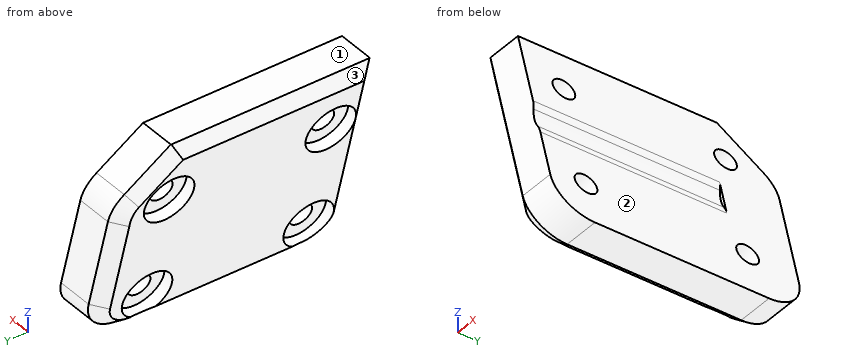
from build123d import *

# Parameters (mm, degrees)
CYLINDER119_R               = 2
CYLINDER119_DEPTH           = 1
CYLINDER119_PLACEMENT_ANGLE = 75
CYLINDER121_R               = 2
CYLINDER121_DEPTH           = 1
CYLINDER121_PLACEMENT_ANGLE = 75
CYLINDER122_R               = 2
CYLINDER122_DEPTH           = 1.4
CYLINDER122_PLACEMENT_ANGLE = 75
CYLINDER120_R               = 2
CYLINDER120_DEPTH           = 1.4
CYLINDER120_PLACEMENT_ANGLE = 75
CYLINDER118_R               = 2.4
CYLINDER118_DEPTH           = 15
CYLINDER118_ROLL_ANGLE      = 90
CYLINDER116_R               = 0.9
CYLINDER116_DEPTH           = 9
CYLINDER116_PLACEMENT_ANGLE = 75
CYLINDER117_R               = 0.9
CYLINDER117_DEPTH           = 9
CYLINDER117_PLACEMENT_ANGLE = 75
CYLINDER115_R               = 0.9
CYLINDER115_DEPTH           = 9
CYLINDER115_PLACEMENT_ANGLE = 75
CYLINDER114_R               = 0.9
CYLINDER114_DEPTH           = 9
CYLINDER114_PLACEMENT_ANGLE = 75
BOX098_W                    = 40
BOX098_H                    = 156
BOX098_DEPTH                = 130
BOX098_PITCH_ANGLE          = -15
BOX099_W                    = 30
BOX099_H                    = 156
BOX099_DEPTH                = 130
BOX099_PITCH_ANGLE          = -15
BOX100_W                    = 10
BOX100_H                    = 20
BOX100_DEPTH                = 16
CHAMFER010_SIZE             = 4
FILLET024_R                 = 3
CHAMFER011_SIZE             = 1
FILLET025_R                 = 2


with BuildPart() as cylinder119:
    # Cylinder119 → Cylinder119 (new body)
    with BuildSketch(Plane.XY):
        Circle(CYLINDER119_R)
    extrude(amount=CYLINDER119_DEPTH)


with BuildPart() as cylinder119_1:
    # Cylinder119 placement: moved
    add(cylinder119.part.moved(Location((509, -34, 102.5))).rotate(Axis((509, -34, 102.5), (0, 1, 0)), CYLINDER119_PLACEMENT_ANGLE))


with BuildPart() as fusion122:
    # Cylinder121 → Cylinder121 (new body)
    with BuildSketch(Plane.XY):
        Circle(CYLINDER121_R)
    extrude(amount=CYLINDER121_DEPTH)


with BuildPart() as fusion122_1:
    # Cylinder121 placement: moved
    add(fusion122.part.moved(Location((509, -21, 102.5))).rotate(Axis((509, -21, 102.5), (0, 1, 0)), CYLINDER121_PLACEMENT_ANGLE))

    # Fusion122: union Cylinder119
    add(cylinder119_1.part)


with BuildPart() as cylinder122:
    # Cylinder122 → Cylinder122 (new body)
    with BuildSketch(Plane.XY):
        Circle(CYLINDER122_R)
    extrude(amount=CYLINDER122_DEPTH)


with BuildPart() as cylinder122_1:
    # Cylinder122 placement: moved
    add(cylinder122.part.moved(Location((509, -34, 102.5))).rotate(Axis((509, -34, 102.5), (0, 1, 0)), CYLINDER122_PLACEMENT_ANGLE))


with BuildPart() as fusion123:
    # Cylinder120 → Cylinder120 (new body)
    with BuildSketch(Plane.XY):
        Circle(CYLINDER120_R)
    extrude(amount=CYLINDER120_DEPTH)


with BuildPart() as fusion123_1:
    # Cylinder120 placement: moved
    add(fusion123.part.moved(Location((509, -21, 102.5))).rotate(Axis((509, -21, 102.5), (0, 1, 0)), CYLINDER120_PLACEMENT_ANGLE))

    # Fusion124: union Cylinder122
    add(cylinder122_1.part)


with BuildPart() as fusion123_2:
    # Fusion124 placement: moved
    add(fusion123_1.part.moved(Location((2, 0, -9))))

    # Fusion123: union Fusion122
    add(fusion122_1.part)


with BuildPart() as cylinder118:
    # Cylinder118 → Cylinder118 (new body)
    with BuildSketch(Plane.XY):
        Circle(CYLINDER118_R)
    extrude(amount=CYLINDER118_DEPTH)


with BuildPart() as cylinder118_1:
    # Cylinder118 roll: moved
    add(cylinder118.part.rotate(Axis((0, 0, 0), (1, 0, 0)), CYLINDER118_ROLL_ANGLE))


with BuildPart() as cylinder118_2:
    # Cylinder118 placement: moved
    add(cylinder118_1.part.moved(Location((516, -22, 100))))


with BuildPart() as cylinder116:
    # Cylinder116 → Cylinder116 (new body)
    with BuildSketch(Plane.XY):
        Circle(CYLINDER116_R)
    extrude(amount=CYLINDER116_DEPTH)


with BuildPart() as cylinder116_1:
    # Cylinder116 placement: moved
    add(cylinder116.part.moved(Location((509, -34, 102.5))).rotate(Axis((509, -34, 102.5), (0, 1, 0)), CYLINDER116_PLACEMENT_ANGLE))


with BuildPart() as fusion120:
    # Cylinder117 → Cylinder117 (new body)
    with BuildSketch(Plane.XY):
        Circle(CYLINDER117_R)
    extrude(amount=CYLINDER117_DEPTH)


with BuildPart() as fusion120_1:
    # Cylinder117 placement: moved
    add(fusion120.part.moved(Location((509, -21, 102.5))).rotate(Axis((509, -21, 102.5), (0, 1, 0)), CYLINDER117_PLACEMENT_ANGLE))

    # Fusion120: union Cylinder116
    add(cylinder116_1.part)


with BuildPart() as cylinder115:
    # Cylinder115 → Cylinder115 (new body)
    with BuildSketch(Plane.XY):
        Circle(CYLINDER115_R)
    extrude(amount=CYLINDER115_DEPTH)


with BuildPart() as cylinder115_1:
    # Cylinder115 placement: moved
    add(cylinder115.part.moved(Location((509, -34, 102.5))).rotate(Axis((509, -34, 102.5), (0, 1, 0)), CYLINDER115_PLACEMENT_ANGLE))


with BuildPart() as fusion121:
    # Cylinder114 → Cylinder114 (new body)
    with BuildSketch(Plane.XY):
        Circle(CYLINDER114_R)
    extrude(amount=CYLINDER114_DEPTH)


with BuildPart() as fusion121_1:
    # Cylinder114 placement: moved
    add(fusion121.part.moved(Location((509, -21, 102.5))).rotate(Axis((509, -21, 102.5), (0, 1, 0)), CYLINDER114_PLACEMENT_ANGLE))

    # Fusion119: union Cylinder115
    add(cylinder115_1.part)


with BuildPart() as fusion121_2:
    # Fusion119 placement: moved
    add(fusion121_1.part.moved(Location((2, 0, -9))))

    # Fusion121: union Fusion120
    add(fusion120_1.part)


with BuildPart() as cube070:
    # Box098 → Box098 (new body)
    with BuildSketch(Plane.XY):
        with Locations((20, 78)):
            Rectangle(BOX098_W, BOX098_H)
    extrude(amount=BOX098_DEPTH)


with BuildPart() as cube070_1:
    # Box098 pitch: moved
    add(cube070.part.rotate(Axis((0, 0, 0), (0, 1, 0)), BOX098_PITCH_ANGLE))


with BuildPart() as cube070_2:
    # Box098 placement: moved
    add(cube070_1.part.moved(Location((569, -38, -9))))


with BuildPart() as fusion118:
    # Box099 → Box099 (new body)
    with BuildSketch(Plane.XY):
        with Locations((15, 78)):
            Rectangle(BOX099_W, BOX099_H)
    extrude(amount=BOX099_DEPTH)


with BuildPart() as fusion118_1:
    # Box099 pitch: moved
    add(fusion118.part.rotate(Axis((0, 0, 0), (0, 1, 0)), BOX099_PITCH_ANGLE))


with BuildPart() as fusion118_2:
    # Box099 placement: moved
    add(fusion118_1.part.moved(Location((533.4, -38, -7))))

    # Fusion118: union Cube070
    add(cube070_2.part)


with BuildPart() as fusion118_3:
    # Fusion118 placement: moved
    add(fusion118_2.part.moved(Location((-22, 0, 0))))


with BuildPart() as door_rear_bar_holder_left:
    # Box100 → Box100 (new body)
    with BuildSketch(Plane(origin=(511, -37, 98), x_dir=(1, 0, 0), z_dir=(0, 0, 1))):
        with Locations((5, 10)):
            Rectangle(BOX100_W, BOX100_H)
    extrude(amount=BOX100_DEPTH)

    # Chamfer010
    chamfer010_edges = [door_rear_bar_holder_left.edges().sort_by_distance(p)[0] for p in [
        (516, -17, 114),
    ]]
    chamfer(chamfer010_edges, length=CHAMFER010_SIZE)


with BuildPart() as door_rear_bar_holder_left_1:
    # Chamfer010 placement: moved
    add(door_rear_bar_holder_left.part.moved(Location((0, 0, -7))))

    # Cut117: cut Fusion118
    add(fusion118_3.part, mode=Mode.SUBTRACT)


with BuildPart() as door_rear_bar_holder_left_2:
    # Cut117 placement: moved
    add(door_rear_bar_holder_left_1.part.moved(Location((-4, 0, 0))))

    # Cut118: cut Fusion121
    add(fusion121_2.part, mode=Mode.SUBTRACT)

    # Fillet024
    fillet024_edges = [door_rear_bar_holder_left_2.edges().sort_by_distance(p)[0] for p in [
        (510.986782, -17, 103),
        (514.202173, -37, 91),
        (514.202173, -17, 91),
    ]]
    fillet(fillet024_edges, radius=FILLET024_R)

    # Chamfer011
    chamfer011_edges = [door_rear_bar_holder_left_2.edges().sort_by_distance(p)[0] for p in [
        (507.912077, -29, 107),
        (512.199265, -27, 91),
    ]]
    chamfer(chamfer011_edges, length=CHAMFER011_SIZE)

    # Cut119: cut Cylinder118
    add(cylinder118_2.part, mode=Mode.SUBTRACT)

    # Fillet025
    fillet025_edges = [door_rear_bar_holder_left_2.edges().sort_by_distance(p)[0] for p in [
        (514.226943, -29.5, 98.382512),
        (513.655743, -29.5, 100.514257),
    ]]
    fillet(fillet025_edges, radius=FILLET025_R)

    # Cut120: cut Fusion123
    add(fusion123_2.part, mode=Mode.SUBTRACT)


solid = door_rear_bar_holder_left_2.part
Work out the finished part from the listing and answer in its coordinate system (mm). Face numbers are marked on the shaded views. Round coordinates to 2 decimals unless told otherwise and drop trailing zeros. Order: outer loops, then holes, each group sorted by start corner. A loop starts at its lowest first (then second) coordinate and runs counter-clockwise, first axis right, second up. Notation, with made-up numbers: M 50,-30.75 L 87,-30.75 A20 ccw 87,-10.75 Z; hole C 66.5,30 d11. An arc over 180 degrees is marked long. One line per item, written item: value.
Q1. Flat-ended cylindrical pins translate along their axes: pin 1 (1 mm diameter, centred on y = -30, z = 102.5, fed in from -X); pin 2 (2 mm diameter, centred on y = -25, z = 100.5, fed in from -X). Find the tip coordinate at first contact, or state that the pin passes through.
Derived:
pin 1: x = 508.98
pin 2: x = 509.39
Q2. Determine the mould class of the marked faces 1, 2 and 3 for opening direction X: released by +X, released by -X, zero draft, split by the parting line, or undercut.
Derived:
face 1: zero draft
face 2: released by +X
face 3: released by -X
Q3. Find section B-B on y = -27. Write down the section's boundary in (x, z), then the cut area to 3 significant figures.
Derived:
outline: M 508.17,106.03 L 511.94,91.97 L 513.2,91 L 516.21,91 L 514.33,97.99 A2 ccw 514.04,98.62 A2.4 cw 513.61,100.21 A2 ccw 513.55,100.91 L 511.92,107 L 508.91,107 Z
area: 62.7 mm²
Q4. Straight lines are drawn through the part: line 1 (Y direction, x = 511.5, z = 105); line 2 (Z direction, x = 513, y = -34.5); line 3 (Y direction, x = 510.5, z = 104.25). For each, find the intervals that lie inside material, in ascending order.
Derived:
line 1: -37 to -19
line 2: 91.19 to 93.26, 94.81 to 102.8
line 3: -37 to -18.25
